from build123d import *

# Parameters (mm, degrees)
F0_R     = 3.175
F0_R_2   = 31.877
F1_DEPTH = 4.7752


with BuildPart() as f1:
    # F0 (on Front) → F1 (new body)
    with BuildSketch(Plane.XZ):
        with BuildLine():
            Line((444.5, 180.975), (-190.5, 180.975))
            ThreePointArc((-190.5, 180.975), (-370.105122, 106.580122), (-444.5, -73.025))
            Line((-444.5, -73.025), (-444.5, -180.975))
            Line((-444.5, -180.975), (444.5, -180.975))
            Line((444.5, -180.975), (444.5, 180.975))
        make_face()
        with Locations((-425.45, -161.925)):
            Circle(F0_R, mode=Mode.SUBTRACT)
        with Locations((-323.85, -104.775)):
            Circle(F0_R_2, mode=Mode.SUBTRACT)
        with Locations((-212.725, -161.925)):
            Circle(F0_R, mode=Mode.SUBTRACT)
        with Locations((-171.45, -104.775)):
            Circle(F0_R_2, mode=Mode.SUBTRACT)
        with Locations((-19.05, -104.775)):
            Circle(F0_R_2, mode=Mode.SUBTRACT)
        with Locations((-425.45, -73.025)):
            Circle(F0_R, mode=Mode.SUBTRACT)
        with Locations((0, -161.925)):
            Circle(F0_R, mode=Mode.SUBTRACT)
        with Locations((212.725, -161.925)):
            Circle(F0_R, mode=Mode.SUBTRACT)
        with Locations((133.35, -104.775)):
            Circle(F0_R_2, mode=Mode.SUBTRACT)
        with Locations((425.45, -161.925)):
            Circle(F0_R, mode=Mode.SUBTRACT)
        with Locations((-323.85, 47.625)):
            Circle(F0_R_2, mode=Mode.SUBTRACT)
        with Locations((-171.45, 47.625)):
            Circle(F0_R_2, mode=Mode.SUBTRACT)
        with Locations((-19.05, 47.625)):
            Circle(F0_R_2, mode=Mode.SUBTRACT)
        with Locations((133.35, 47.625)):
            Circle(F0_R_2, mode=Mode.SUBTRACT)
        with Locations((425.45, 0)):
            Circle(F0_R, mode=Mode.SUBTRACT)
        with Locations((425.45, 161.925)):
            Circle(F0_R, mode=Mode.SUBTRACT)
    extrude(amount=F1_DEPTH)


solid = f1.part
The model under review builds one solid part; all positions refer to its coordinate system, in mm. Round coordinates to 2 decimals unless told otherwise and drop trailing zeros. Loops run counter-clockwise (first coordinate to the right, second up) from the corner with the lowest first, then second, coordinate; pieces in that order, holes last. Notation, with made-up numbers: (-14, -18) -> (0, -18) arc R19 cw to (0, 10) -> close; hole circle Ø4 at (69, 8.5). An arc over 180 degrees is marked (long way). Write item = value, one per line. Start each with the question number.
Item 1: Take a section at A-A on x = -19.05. Give the boundary of the cut face in (y, z) (3 decimals).
Item 2: Mouldability with a two-part tool opening along X and no side actions: class faces 1 (the cylindrical face through (162.8, -2.35, 35.42)), 2 (the cylindrical face through (-368.119, -2.354, 108.544)), 3 (the cylindrical face through (-355.696, -2.354, -103.373)), 4 (the flat face through (-6, 0, 3)) as released by +X, released by -X, zero draft, split by the parting line, or undercut.
Item 3: To check wall thickness, follow L1, parallel to Z at x = -17.5, y = -4.15 (3 decimals); L2, parallel to Z at x = 425.45, y = -3 (3 decimals); L3, parallel to X at y = -2.7, z = -112. State the ranges of each line that lie inside material, in increasing order.
Item 4: Take a section at C-C on y = -2.25. Count the separate pieces of the cut face and the enclosed holes in it, plus the area to 3 significant figures.
Item 5: Take a section at B-B on z = -125. Give the boundary of the cut face in (x, y).
Item 6: Insertion check: pin 1 (7.5 mm diameter, centred on x = 0, z = -161.925, fed in from +Y); pin 2 (2 mm diameter, centred on y = -1, z = -36, fed in from -X). Each pin has a flat end and moves straight along its axis. Give the tip position at first contact, or say it passes through.
Item 7: Take a section at D-D on x = -175. Give the boundary of the cut face in (y, z) (3 decimals).
Result:
q1.outline = (-4.775, -180.975) -> (0, -180.975) -> (0, -136.652) -> (-4.775, -136.652) -> close; (-4.775, -72.898) -> (0, -72.898) -> (0, 15.748) -> (-4.775, 15.748) -> close; (-4.775, 79.502) -> (0, 79.502) -> (0, 180.975) -> (-4.775, 180.975) -> close
q2.face_1 = undercut
q2.face_2 = released by -X
q2.face_3 = undercut
q2.face_4 = zero draft
q3.L1 = -180.975 to -136.614, -72.936 to 15.786, 79.464 to 180.975
q3.L2 = -180.975 to -165.1, -158.75 to -3.175, 3.175 to 158.75, 165.1 to 180.975
q3.L3 = -444.5 to -354.9, -292.8 to -202.5, -140.4 to -50.1, 12 to 102.3, 164.4 to 444.5
q4.separate_pieces = 1
q4.enclosed_holes = 16
q4.area = 282,000 mm²
q5.outline = (-444.5, -4.78) -> (-348.49, -4.78) -> (-348.49, 0) -> (-444.5, 0) -> close; (-299.21, -4.78) -> (-196.09, -4.78) -> (-196.09, 0) -> (-299.21, 0) -> close; (-146.81, -4.78) -> (-43.69, -4.78) -> (-43.69, 0) -> (-146.81, 0) -> close; (5.59, -4.78) -> (108.71, -4.78) -> (108.71, 0) -> (5.59, 0) -> close; (157.99, -4.78) -> (444.5, -4.78) -> (444.5, 0) -> (157.99, 0) -> close
q6.pin_1 = 0
q6.pin_2 = -441.93
q7.outline = (-4.775, -180.975) -> (0, -180.975) -> (0, -136.454) -> (-4.775, -136.454) -> close; (-4.775, -73.096) -> (0, -73.096) -> (0, 15.946) -> (-4.775, 15.946) -> close; (-4.775, 79.304) -> (0, 79.304) -> (0, 180.975) -> (-4.775, 180.975) -> close
